The listing builds one solid part. Answer for the finished solid, in the listing's coordinates (mm). Face numbers are marked on the shaded views. Round coordinates to 2 decimals unless told otherwise and drop trailing zeros. Write each loop counter-clockwise with the first axis right and the second up, starting at its lowest first coordinate (ties: lowest second). Pieces come first, ordered by that corner, then holes. Notation, with made-up numbers: M 18.5,8.25 L 53.5,8.25 A21 ccw 53.5,44.25 Z; hole C 44,-5.5 d11. An arc over 180 degrees is marked long. Write each question's results on one line, items separated by ' | '.
from build123d import *

# Parameters (mm, degrees)
SKETCH1_R           = 98.425
SKETCH1_R_2         = 9.525
BOSS_EXTRUDE1_DEPTH = 7.62
BOSS_EXTRUDE2_DEPTH = 25.4
SKETCH5_R           = 5.2578
CUT_EXTRUDE3_DEPTH  = 19.05
SKETCH6_R           = 3.175
CUT_EXTRUDE4_DEPTH  = 12.7
CIRPATTERN1_COUNT   = 12
CIRPATTERN2_COUNT   = 4
SKETCH8_R           = 1.7526
CUT_EXTRUDE6_DEPTH  = 34.02
CIRPATTERN3_COUNT   = 4


with BuildPart() as part:
    # Sketch1 → Boss-Extrude1 (new body)
    with BuildSketch(Plane(origin=(0, 0, 0), x_dir=(1, 0, 0), z_dir=(0, 1, 0))):
        Circle(SKETCH1_R)
        Circle(SKETCH1_R_2, mode=Mode.SUBTRACT)
    extrude(amount=BOSS_EXTRUDE1_DEPTH)

    # Sketch2 → Boss-Extrude2 (add)
    with BuildSketch(Plane.XZ):
        with BuildLine():
            Line((-14.092921054, 83.751577801), (-14.875155352, 97.29445194))
            ThreePointArc((-14.875155352, 97.29445194), (-0.679076319, 98.422657353), (13.531218764, 97.490444372))
            Line((13.531218764, 97.490444372), (13.333659481, 80.753245397))
            ThreePointArc((13.333659481, 80.753245397), (-1.546485964, 71.578862712), (-14.092921054, 83.751577801))
        make_face()
        with BuildLine():
            Line((83.751577801, 14.092921054), (97.29445194, 14.875155352))
            ThreePointArc((97.29445194, 14.875155352), (98.422657353, 0.679076319), (97.490444372, -13.531218764))
            Line((97.490444372, -13.531218764), (80.753245397, -13.333659481))
            ThreePointArc((80.753245397, -13.333659481), (71.578862712, 1.546485964), (83.751577801, 14.092921054))
        make_face()
        with BuildLine():
            Line((14.092921054, -83.751577801), (14.875155352, -97.29445194))
            ThreePointArc((14.875155352, -97.29445194), (0.679076319, -98.422657353), (-13.531218764, -97.490444372))
            Line((-13.531218764, -97.490444372), (-13.333659481, -80.753245397))
            ThreePointArc((-13.333659481, -80.753245397), (1.546485964, -71.578862712), (14.092921054, -83.751577801))
        make_face()
        with BuildLine():
            Line((-83.751577801, -14.092921054), (-97.29445194, -14.875155352))
            ThreePointArc((-97.29445194, -14.875155352), (-98.422657353, -0.679076319), (-97.490444372, 13.531218764))
            Line((-97.490444372, 13.531218764), (-80.753245397, 13.333659481))
            ThreePointArc((-80.753245397, 13.333659481), (-71.578862712, -1.546485964), (-83.751577801, -14.092921054))
        make_face()
    extrude(amount=BOSS_EXTRUDE2_DEPTH)

    # Sketch5 → Cut-Extrude3 (cut)
    with BuildSketch(Plane.XZ.offset(25.4)):
        with Locations((0, 85.725)):
            Circle(SKETCH5_R)
    cut_extrude3 = extrude(amount=-CUT_EXTRUDE3_DEPTH, mode=Mode.SUBTRACT)

    # Sketch6 → Cut-Extrude4 (cut)
    with BuildSketch(Plane(origin=(0, 7.62, 0), x_dir=(1, 0, 0), z_dir=(0, 1, 0))):
        with Locations((-23.830763578, 88.937620456)):
            Circle(SKETCH6_R)
    cut_extrude4 = extrude(amount=-CUT_EXTRUDE4_DEPTH, mode=Mode.SUBTRACT)

    # CirPattern1: Cut-Extrude4 ×12 about axis
    cirpattern1_axis = Axis((0, 0, 0), (0, 1, 0))
    for i in range(1, CIRPATTERN1_COUNT):
        add(cut_extrude4.rotate(cirpattern1_axis, i * 360 / CIRPATTERN1_COUNT), mode=Mode.SUBTRACT)

    # CirPattern2: Cut-Extrude3 ×4 about axis
    cirpattern2_axis = Axis((0, 0, 0), (0, 1, 0))
    for i in range(1, CIRPATTERN2_COUNT):
        add(cut_extrude3.rotate(cirpattern2_axis, i * 360 / CIRPATTERN2_COUNT), mode=Mode.SUBTRACT)

    # Sketch8 → Cut-Extrude6 (cut, through all)
    with BuildSketch(Plane(origin=(0, 7.62, 0), x_dir=(1, 0, 0), z_dir=(0, 1, 0))):
        with Locations((0, 85.725)):
            Circle(SKETCH8_R)
    cut_extrude6 = extrude(amount=-CUT_EXTRUDE6_DEPTH, mode=Mode.SUBTRACT)

    # CirPattern3: Cut-Extrude6 ×4 about axis
    cirpattern3_axis = Axis((0, 0, 0), (0, 1, 0))
    for i in range(1, CIRPATTERN3_COUNT):
        add(cut_extrude6.rotate(cirpattern3_axis, i * 360 / CIRPATTERN3_COUNT), mode=Mode.SUBTRACT)


solid = part.part
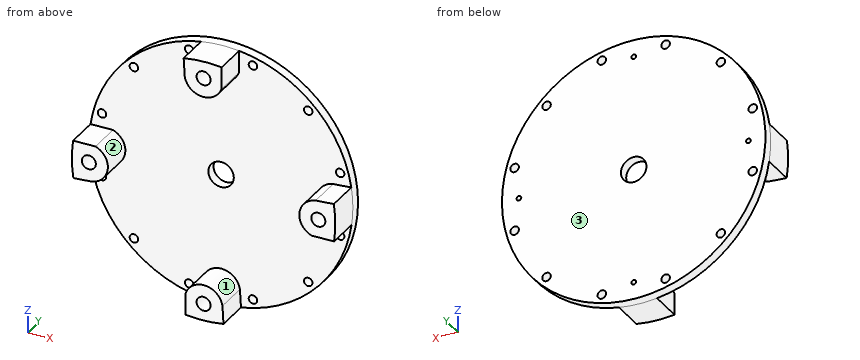
1) Section C-C (x = 46) is taken. Determine the outline of the cut face in (y, z), then the cut area to 3 significant figures.
Return value:
outline: M 0,-87.01 L 7.62,-87.01 L 7.62,87.01 L 0,87.01 Z | area: 1,330 mm²
2) Find the intervals of material crossed by line 1 (X direction, y = -12, z = 0) (3 decimals); line 2 (Z direction, x = 0, y = 2) (3 decimals); line 3 (Z direction, x = -65.5, y = 0.5), in increasing order.
Return value:
line 1: -98.425 to -90.983, -80.467 to -71.495, 71.495 to 80.467, 90.983 to 98.425 | line 2: -98.425 to -87.478, -83.972 to -9.525, 9.525 to 83.972, 87.478 to 98.425 | line 3: -73.47 to -68.26, -61.96 to 61.96, 68.26 to 73.47
3) Each of these flat-tipped pins is pushed along its axis until it touches: pin 1 (10 mm diameter, centred on x = -88.94, z = 23.83, fed in from +Y); pin 2 (8 mm diameter, centred on y = -0.5, z = 68.5, fed in from -X); pin 3 (8 mm diameter, centred on x = 64.5, z = 62.5, fed in from -Y); pin 4 (8.5 mm diameter, centred on x = 85.725, z = 0, fed in from -Y). Where does it stop, or does it pass through?
Return value:
pin 1: y = 7.62 | pin 2: x = -74.32 | pin 3: y = 0 | pin 4: y = -6.35
4) Section A-A (y = -11.5) is taken. Determine the outline of the cut face in (x, z) (3 decimals).
Return value:
outline: M -97.49,13.531 A98.425 ccw -97.294,-14.875 L -83.752,-14.093 A14.23 ccw -80.753,13.334 Z; M -14.875,97.294 L -14.093,83.752 A14.23 ccw 13.334,80.753 L 13.531,97.49 A98.425 ccw Z; M -13.531,-97.49 A98.425 ccw 14.875,-97.294 L 14.093,-83.752 A14.23 ccw -13.334,-80.753 Z; M 80.753,-13.334 L 97.49,-13.531 A98.425 ccw 97.294,14.875 L 83.752,14.093 A14.23 ccw Z; hole C -85.725,0 d10.516; hole C 0,-85.725 d10.516; hole C 0,85.725 d10.516; hole C 85.725,0 d10.516
5) The mould has two halves that part along X. Classify the marked faces 1, 2 and 3: +X half, -X half, draft (parallel to the pull), parting line (faces both ways), or undercut.
Return value:
face 1: parting line | face 2: undercut | face 3: draft
6) Section B-B (y = 3.5) is taken. State how many separate pieces and enclosed holes the cut face has, then the cut area to 3 significant figures.
Return value:
separate pieces: 1 | enclosed holes: 17 | area: 29,700 mm²
7) Section D-D (z = -51.5) is taken. Determine the outline of the cut face in (x, y), then the cut area to 3 significant figures.
Return value:
outline: M -83.88,0 L 83.88,0 L 83.88,7.62 L -83.88,7.62 Z | area: 1,280 mm²
